Design review of the part shown in the three views and the two pictorial views. Dimensions are in mm from the part's minimum x, y and z. A direction names the side the tool comes from. Coordinates: 2 decimals unless noted, no trailing zeros. Loops run counter-clockwise (first coordinate to the right, second up) from the corner with the lowest first, then second, coordinate; pieces in that order, holes last. Notation, with made-up numbers: M -33.5,65.5 L 24.5,65.5 A18 ccw 24.5,90.5 Z; hole C 64.5,68.5 d11. An arc over 180 degrees is marked long. Write item = value, one per line. Start each with the question number.
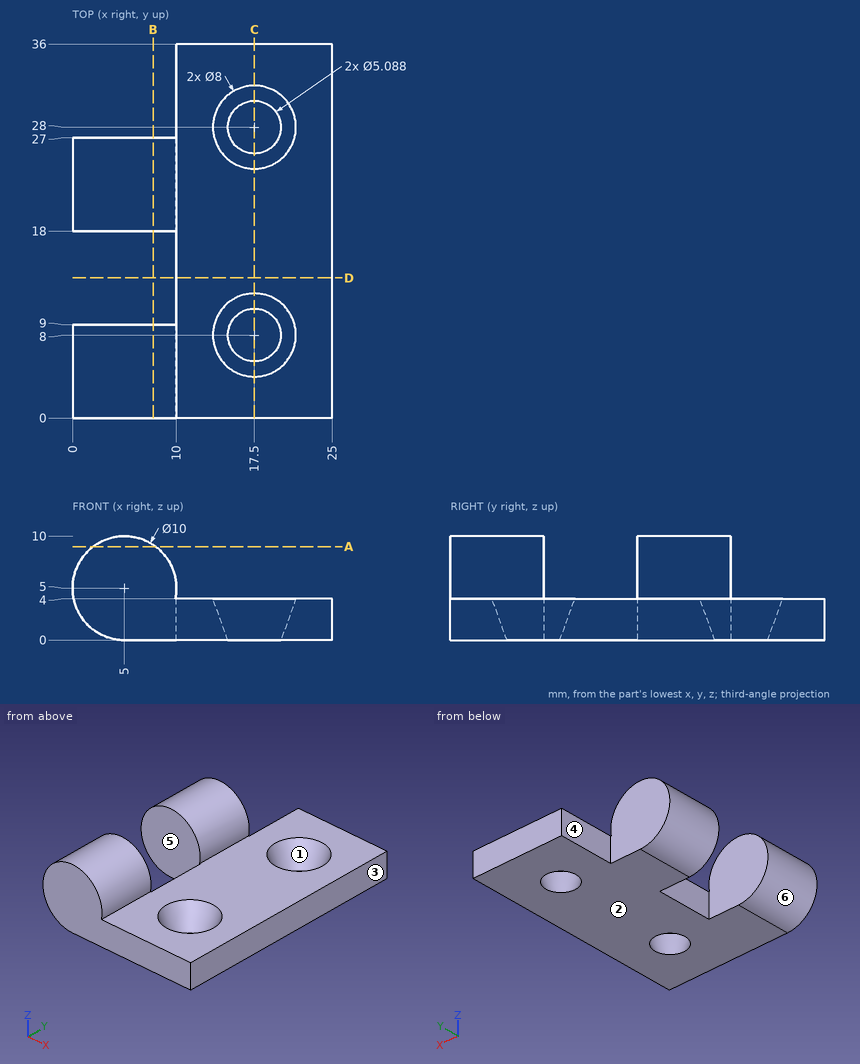
(1) Insertion check: pin 1 (1.5 mm diameter, centred on y = 9.5, z = 1.5, fed in from -X); pin 2 (8 mm diameter, centred on x = 15, y = 25.5, fed in from +Z); pin 3 (4.5 mm diameter, centred on y = 31.5, z = 2, fed in from -X). Each pin has a flat end and moves straight along its axis. Give the tip position at first contact, or say it passes through.
(2) Take a section at A-A (z = 9). State the section outline as (x, y) points.
(3) To check wall thickness, follow L1, parallel to Y at x = 6.5, z = 5.75; L2, parallel to Z at x = 6, y = 4; L3, parallel to Y at x = 15, z = 1 (1 decimal). State the ranges of each line that lie inside material, in increasing order.
(4) Tool access review of the marked faces 4, 5 and 6: name each direction out of +Z, -Z, +X, -X, +Y, -Y from which nothing blocks a thin tool from reaching the whole face with its end or side.
(5) Take a section at B-B (x = 7.75). State the section outline as (y, z) points, plus the area to 3 significant figures.
(6) Take a section at C-C (x = 17.5). State the section outline as (y, z) points.
(7) Take a section at D-D (y = 13.5). State the section outline as (x, z) points.
(8) Mouldability with a two-part tool opening along X and no side actions: class the marked faces 1, 2 and 3 as +X half, -X half, draft (parallel to the pull), parting line (faces both ways), or undercut.
Results list:
q1.pin_1 = 0.96
q1.pin_2 = 4
q1.pin_3 = 10
q2.outline = M 2,0 L 8,0 L 8,9 L 2,9 Z; M 2,18 L 8,18 L 8,27 L 2,27 Z
q3.L1 = 0 to 9, 18 to 27
q3.L2 = 0 to 9.9
q3.L3 = 0 to 6.5, 9.5 to 26.5, 29.5 to 36
q4.face_4 = +Z, -Z, -X, +Y
q4.face_5 = +Z, -Z, -X
q4.face_6 = +Y, -Y
q5.outline = M 0,0 L 9,0 L 9,9.18 L 0,9.18 Z; M 18,0 L 27,0 L 27,9.18 L 18,9.18 Z
q5.area = 165 mm^2
q6.outline = M 0,0 L 5.46,0 L 4,4 L 0,4 Z; M 10.54,0 L 25.46,0 L 24,4 L 12,4 Z; M 30.54,0 L 36,0 L 36,4 L 32,4 Z
q7.outline = M 10,0 L 25,0 L 25,4 L 10,4 Z
q8.face_1 = undercut
q8.face_2 = draft
q8.face_3 = +X half
